Autodesk Inventor part; units mm, degrees
ref_plane "YZ Plane" through (0, 0, 0) normal (1, 0, 0) x (0, 1, 0)
ref_plane "XZ Plane" through (0, 0, 0) normal (0, 1, 0) x (-1, 0, 0)
ref_plane "XY Plane" through (0, 0, 0) normal (0, 0, 1) x (1, 0, 0)
sketch "Sketch1" plane through (0, 0, 0) normal (0, 1, 0) x (-1, 0, 0)
  line L0 (0, 0) -> (0, -40) construction
  line L1 (-1.65, 0) -> (-1.65, -40)
  line L2 (1.65, -40) -> (1.65, 0)
  arc A0 (1.65, 0) -> (-1.65, 0) centre (0, 0) ccw
  arc A1 (-1.65, -40) -> (1.65, -40) centre (0, -40) ccw
  line L3 (-5, 20) -> (7.65, 20)
  line L4 (7.65, 20) -> (7.65, -60)
  line L5 (7.65, -60) -> (-5, -60)
  line L6 (-5, -60) -> (-5, 20)
  circle A2 centre (0, -40) radius 5
  circle A3 centre (0, 0) radius 5
  point P0 (0, -20)
  dimension "d0" = 3.3
  dimension "d1" = 40
  dimension "d2" = 10
  dimension "d3" = 10
  dimension "d4" = 20
  dimension "d5" = 20
  dimension "d6" = 6
extrude "Extrusion1" add sketch "Sketch1" along normal blind 8 contours L1 A3 L2 A0 | L1 A2 L6 A3 | L1 A1 L2 A2 | L6 L3 L4 L5 A2 L2 A3 picked at (-2.0178, -2.9645) picked at (-2.0178, -37.0355)
ref_plane "Work Plane1" through (0, 0, 0) normal (1, 0, 0) x (0, 0, -1)
properties part number "Rail"
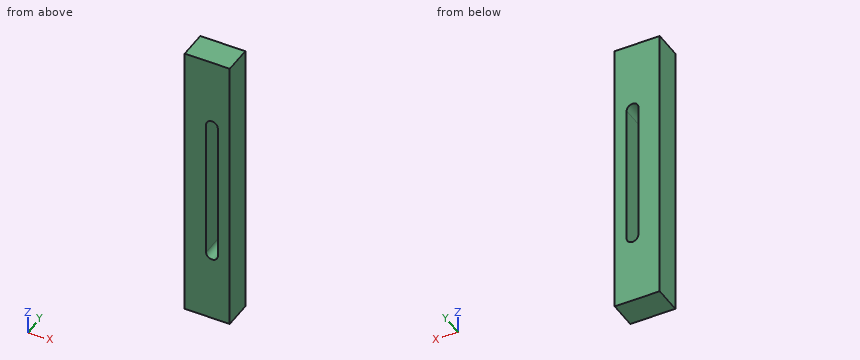
Design review of the part built by this model. Coordinates are the model's own, in mm. Coordinates: 2 decimals unless noted, no trailing zeros. Order: outer loops, then holes, each group sorted by start corner. A loop starts at its lowest first (then second) coordinate and runs counter-clockwise, first axis right, second up.
1) Take a section at A-A, the plane x = 0. Give the boundary of the cut face in (y, z).
2) Take a section at B-B, the plane y = 2. Give the boundary of the cut face in (x, z).
3) Wall thickness on line 1 along X through (y, z) = (2, -34); line 2 along Z through (x, y) = (-1.25, 5.25); line 3 along X through (y, z) = (7.5, -41.5): over which ranges is each line inside the solid? List them lowest first.
Returned:
1. outline: (0, -60) - (8, -60) - (8, -41.65) - (0, -41.65) - close; (0, 1.65) - (8, 1.65) - (8, 20) - (0, 20) - close
2. outline: (-7.65, -60) - (5, -60) - (5, 20) - (-7.65, 20) - close; hole (-1.65, -40) arc R1.65 ccw to (1.65, -40) - (1.65, 0) arc R1.65 ccw to (-1.65, 0) - close
3. line 1: x = -7.65 to -1.65, 1.65 to 5
3. line 2: z = -60 to -41.08, 1.08 to 20
3. line 3: x = -7.65 to -0.69, 0.69 to 5
